```python
from build123d import *

# Parameters (mm, degrees)
SKETCH1_W           = 60
SKETCH1_H           = 60
SKETCH1_R           = 2
BOSS_EXTRUDE1_DEPTH = 6
SKETCH2_R           = 12
BOSS_EXTRUDE2_DEPTH = 6
SKETCH3_R           = 4
BOSS_EXTRUDE3_DEPTH = 20
CUT_EXTRUDE1_START  = -19
CUT_EXTRUDE1_DEPTH  = 19
SKETCH5_R           = 30
BOSS_EXTRUDE4_DEPTH = 27
SKETCH6_R           = 22.5
BOSS_EXTRUDE5_DEPTH = 30
SKETCH7_R           = 21
BOSS_EXTRUDE6_DEPTH = 43


with BuildPart() as part:
    # Sketch1 → Boss-Extrude1 (new body)
    with BuildSketch(Plane.XY):
        Rectangle(SKETCH1_W, SKETCH1_H)
        with Locations((-25, 25)):
            Circle(SKETCH1_R, mode=Mode.SUBTRACT)
        with Locations((25, 25)):
            Circle(SKETCH1_R, mode=Mode.SUBTRACT)
        with Locations((-25, -25)):
            Circle(SKETCH1_R, mode=Mode.SUBTRACT)
        with Locations((25, -25)):
            Circle(SKETCH1_R, mode=Mode.SUBTRACT)
    extrude(amount=BOSS_EXTRUDE1_DEPTH)

    # Sketch2 → Boss-Extrude2 (add)
    with BuildSketch(Plane.XY.offset(6)):
        Circle(SKETCH2_R)
    extrude(amount=BOSS_EXTRUDE2_DEPTH)

    # Sketch3 → Boss-Extrude3 (add)
    with BuildSketch(Plane.XY.offset(12)):
        Circle(SKETCH3_R)
    extrude(amount=BOSS_EXTRUDE3_DEPTH)

    # Sketch4 → Cut-Extrude1 (cut)
    with BuildSketch(Plane.XY.offset(32).offset(CUT_EXTRUDE1_START)):
        with BuildLine():
            Line((-2.645751311, 3), (2.645751311, 3))
            ThreePointArc((2.645751311, 3), (0, 4), (-2.645751311, 3))
        make_face()
    extrude(amount=CUT_EXTRUDE1_DEPTH, mode=Mode.SUBTRACT)

    # Sketch5 → Boss-Extrude4 (add)
    with BuildSketch(Plane(origin=(0, 0, 0), x_dir=(-1, 0, 0), z_dir=(0, 0, -1))):
        Circle(SKETCH5_R)
    extrude(amount=BOSS_EXTRUDE4_DEPTH)

    # Sketch6 → Boss-Extrude5 (add)
    with BuildSketch(Plane(origin=(0, 0, -27), x_dir=(-1, 0, 0), z_dir=(0, 0, -1))):
        Circle(SKETCH6_R)
    extrude(amount=BOSS_EXTRUDE5_DEPTH)

    # Sketch7 → Boss-Extrude6 (add)
    with BuildSketch(Plane(origin=(0, 0, -57), x_dir=(-1, 0, 0), z_dir=(0, 0, -1))):
        Circle(SKETCH7_R)
    extrude(amount=BOSS_EXTRUDE6_DEPTH)


solid = part.part
```
Work out the finished part from the listing and answer in its coordinate system (mm). A direction names the side the tool comes from. Give positions to 0.01 mm unless a question says otherwise; leave off trailing zeros. Order: outer loops, then holes, each group sorted by start corner. A loop starts at its lowest first (then second) coordinate and runs counter-clockwise, first axis right, second up. Notation, with made-up numbers: (-35, 41.5) - (-27, 41.5) arc R24 cw to (-27, 78.5) - close; hole circle Ø10 at (57.25, -27.75). An arc over 180 degrees is marked (long way). One line per item, written item: value. Start each with the question number.
1. Section D-D, the plane x = 9 is taken. Write down the section's boundary in (y, z), then the cut area to 3 significant figures.
2. Section A-A, the plane y = -25 is taken. Write down the section's boundary in (x, z), then the cut area to 3 significant figures.
3. Consider line 1 (Y direction, x = 25, z = 1.6); line 2 (Z direction, x = -11, y = 11); line 3 (Z direction, x = -26, y = 21.5). Determine where each line is inside the solid, lowest interval first.
4. Section C-C, the plane y = -8 is taken. Write down the section's boundary in (x, z).
5. Each of these flat-tipped pins is pushed along its axis until it touches: pin 1 Ø12 at (x, z) = (-14, -14) entering from +Y; pin 2 Ø4 at (y, z) = (12.5, -30) entering from -X; pin 3 Ø3.5 at (x, y) = (25, -25) entering from -Z; pin 4 Ø3 at (x, z) = (-10, -48) entering from +Y. Where does it stop, or does it pass through?
6. Which of the six approach directions +Z, -Z, +X, -X, +Y, -Y give full straight-line access (tool end or side, diameter ignored) to faces 1 (the face through (-23, -23, 0)), 2 (the face through (-14, 0, 6)), 3 (the face through (-10.382, -19.961, -41.79)), 4 (the face through (23, -24, 0)), 5 (the face through (0, 3, 22))?
Filled sheet:
1. outline: (-30, 0) - (-28.62, 0) - (-28.62, -27) - (-20.62, -27) - (-20.62, -57) - (-18.97, -57) - (-18.97, -100) - (18.97, -100) - (18.97, -57) - (20.62, -57) - (20.62, -27) - (28.62, -27) - (28.62, 0) - (30, 0) - (30, 6) - (7.94, 6) - (7.94, 12) - (-7.94, 12) - (-7.94, 6) - (-30, 6) - close
1. area: 4,870 mm²
2. outline: (-30, 0) - (-27, 0) - (-27, 6) - (-30, 6) - close; (-23, 0) - (-16.58, 0) - (-16.58, -27) - (16.58, -27) - (16.58, 0) - (23, 0) - (23, 6) - (-23, 6) - close; (27, 0) - (30, 0) - (30, 6) - (27, 6) - close
2. area: 1,210 mm²
3. line 1: -30 to -27, -23 to 23, 27 to 30
3. line 2: -100 to 6
3. line 3: 0 to 6
4. outline: (-30, 0) - (-28.91, 0) - (-28.91, -27) - (-21.03, -27) - (-21.03, -57) - (-19.42, -57) - (-19.42, -100) - (19.42, -100) - (19.42, -57) - (21.03, -57) - (21.03, -27) - (28.91, -27) - (28.91, 0) - (30, 0) - (30, 6) - (8.94, 6) - (8.94, 12) - (-8.94, 12) - (-8.94, 6) - (-30, 6) - close
5. pin 1: y = 28.91
5. pin 2: x = -19.9
5. pin 3: through
5. pin 4: y = 20.83
6. face 1: -Z, -X, -Y
6. face 2: +Z
6. face 3: -Z
6. face 4: -Z, +X, -Y
6. face 5: +Z, +X, -X, +Y
